For this review, use the dimensioned drawing (mm, ordinates from the lowest corner) and the shaded views. Round coordinates to 2 decimals unless told otherwise and drop trailing zeros. Write each loop counter-clockwise with the first axis right and the second up, starting at its lowest first coordinate (ties: lowest second). Pieces come first, ordered by that corner, then holes.
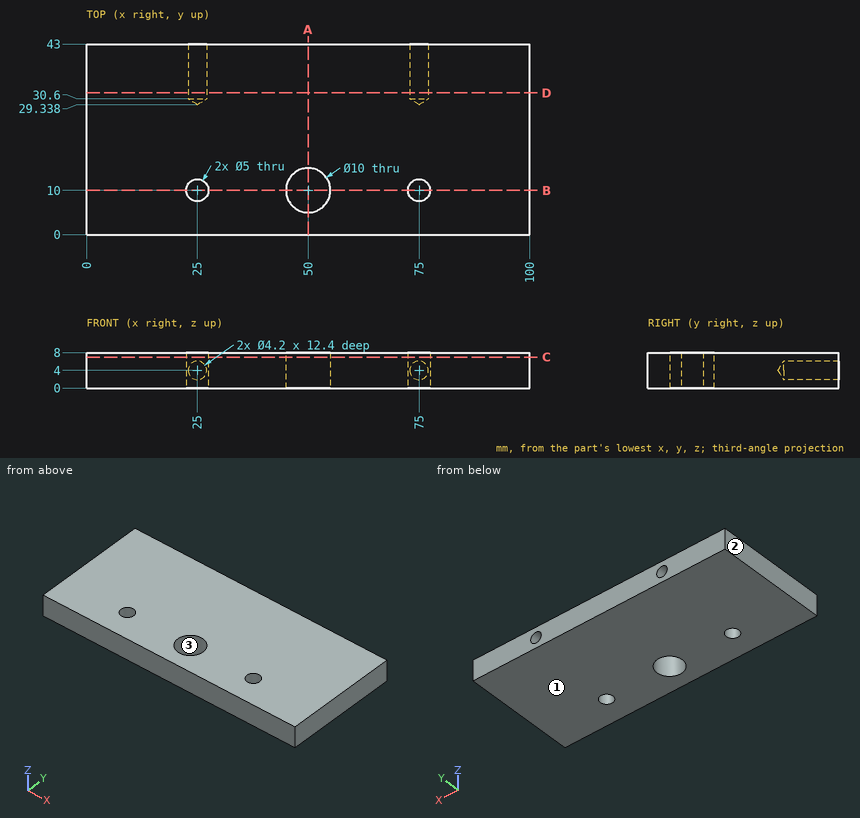
(1) We need section B-B, the plane y = 10. Give the boundary of the cut face in (x, z), and give its area (3 significant figures).
Geometry check:
outline: (0, 0) - (22.5, 0) - (22.5, 8) - (0, 8) - close; (27.5, 0) - (45, 0) - (45, 8) - (27.5, 8) - close; (55, 0) - (72.5, 0) - (72.5, 8) - (55, 8) - close; (77.5, 0) - (100, 0) - (100, 8) - (77.5, 8) - close
area: 640 mm2
(2) We need section C-C, the plane z = 7. Give the boundary of the cut face in (x, y).
Geometry check:
outline: (0, 0) - (100, 0) - (100, 43) - (0, 43) - close; hole circle Ø5 at (25, 10); hole circle Ø10 at (50, 10); hole circle Ø5 at (75, 10)
(3) We need section D-D, the plane y = 32. Give the boundary of the cut face in (x, z), and give its area (3 significant figures).
Geometry check:
outline: (0, 0) - (100, 0) - (100, 8) - (0, 8) - close; hole circle Ø4.2 at (25, 4); hole circle Ø4.2 at (75, 4)
area: 772 mm2
(4) For pin 1 Ø3.5 at (x, z) = (75, 4) entering from +Y; pin 2 Ø11.5 at (x, y) = (50, 10) entering from +Z; pin 3 Ø4 at (x, y) = (75, 10) entering from +Z; pin 4 Ø4 at (x, z) = (25, 4) entering from +Y, all flat-tipped, find the tip position at first contact; note any pin that passes through.
Geometry check:
pin 1: stops at y = 30.39
pin 2: stops at z = 8
pin 3: passes through
pin 4: stops at y = 30.54
(5) We need section A-A, the plane x = 50. Give the boundary of the cut face in (y, z).
Geometry check:
outline: (0, 0) - (5, 0) - (5, 8) - (0, 8) - close; (15, 0) - (43, 0) - (43, 8) - (15, 8) - close
(6) For line 1 along Z through (x, y) = (75, 35); line 2 along X through (y, z) = (11.5, 1); line 3 along X through (y, z) = (34, 3.25), list the stretches that pass through material, from the lowest coordinate up.
Geometry check:
line 1: z = 0 to 1.9, 6.1 to 8
line 2: x = 0 to 23, 27 to 45.23, 54.77 to 73, 77 to 100
line 3: x = 0 to 23.04, 26.96 to 73.04, 76.96 to 100
(7) Mouldability with a two-part tool opening along X and no side actions: class the marked faces 1, 2 and 3 as pulls with the +X half, pulls with the -X half, needs draft (parallel to the pull), parting line crosses it, or undercut.
Geometry check:
face 1: needs draft
face 2: pulls with the -X half
face 3: undercut
